Autodesk Inventor part; units mm, degrees
ref_plane "YZ Plane" through (0, 0, 0) normal (1, 0, 0) x (0, 1, 0)
ref_plane "XZ Plane" through (0, 0, 0) normal (0, 1, 0) x (-1, 0, 0)
ref_plane "XY Plane" through (0, 0, 0) normal (0, 0, 1) x (1, 0, 0)
sketch "Sketch1" plane through (0, 0, 0) normal (0, 0, 1) x (1, 0, 0)
  circle A0 centre (-7.5, 22.4) radius 1.5
  circle A1 centre (-7.5, 3.2) radius 1.5
  circle A2 centre (-18, 3.2) radius 1.5
  circle A3 centre (-18, 22.4) radius 1.5
  line L0 (0, 0) -> (-24, 0)
  line L1 (0, 25.6) -> (0, 0)
  line L2 (-24, 25.6) -> (0, 25.6)
  line L3 (-24, 0) -> (-24, 25.6)
extrude "Extrusion1" add sketch "Sketch1" along normal blind 6
properties part number "yCarBeltTensionerHolder"
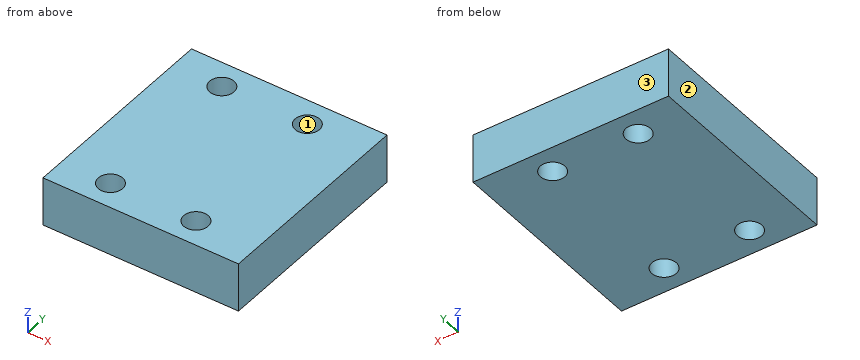
Here's how the part is built. I have some questions about the finished solid (model axes, mm). Face numbers are marked on the shaded views. Round coordinates to 2 decimals unless told otherwise and drop trailing zeros. Order: outer loops, then holes, each group sorted by start corner. A loop starts at its lowest first (then second) coordinate and runs counter-clockwise, first axis right, second up. Notation, with made-up numbers: M -23.5,-26 L 28.5,-26 A25 cw 28.5,-12 Z; hole C 25.5,-15 d3. An arc over 180 degrees is marked long. Use CSV: the item, a comma, the result in double quotes.
1) If we mould it in two halves opening along X, with no side actions, what happens to the marked faces 1, 2 and 3? For each: pulls with the +X half, pulls with the -X half, needs draft (parallel to the pull), parting line crosses it, or undercut.
Taken from the geometry:
face 1,"undercut"
face 2,"pulls with the -X half"
face 3,"needs draft"
2) I want a section at B-B (x = -7.5). List the corners of the cut face in (y, z) for me, then the cut area to 3 significant figures.
Taken from the geometry:
outline,"M 0,0 L 1.7,0 L 1.7,6 L 0,6 Z; M 4.7,0 L 20.9,0 L 20.9,6 L 4.7,6 Z; M 23.9,0 L 25.6,0 L 25.6,6 L 23.9,6 Z"
area,"118 mm^2"
3) I need wall thicknesses on line 1 along Y through (x, z) = (-7.5, 1.8); line 2 along X through (y, z) = (22, 3.95); line 3 along Y through (x, z) = (-8.25, 4.85). Which ranges of each line are inside material? Lowest first, please. Write a range as [from, to].
Taken from the geometry:
line 1,"[0, 1.7], [4.7, 20.9], [23.9, 25.6]"
line 2,"[-24, -19.45], [-16.55, -8.95], [-6.05, 0]"
line 3,"[0, 1.9], [4.5, 21.1], [23.7, 25.6]"
4) I want a section at C-C (y = 22.4). List the corners of the cut face in (x, z) for me, then the cut area to 3 significant figures.
Taken from the geometry:
outline,"M -24,0 L -19.5,0 L -19.5,6 L -24,6 Z; M -16.5,0 L -9,0 L -9,6 L -16.5,6 Z; M -6,0 L 0,0 L 0,6 L -6,6 Z"
area,"108 mm^2"
5) I want a section at A-A (z = 0.8). List the corners of the cut face in (x, y) for me.
Taken from the geometry:
outline,"M -24,0 L 0,0 L 0,25.6 L -24,25.6 Z; hole C -18,3.2 d3; hole C -18,22.4 d3; hole C -7.5,3.2 d3; hole C -7.5,22.4 d3"
